Design review of the part built by this model. Coordinates are the model's own, in mm. Face numbers are marked on the shaded views. A direction names the side the tool comes from. Coordinates: 2 decimals unless noted, no trailing zeros. Loops run counter-clockwise (first coordinate to the right, second up) from the corner with the lowest first, then second, coordinate; pieces in that order, holes last. Notation, with made-up numbers: M -13.5,35.25 L 44.5,35.25 A24 ccw 44.5,60.25 Z; hole C 3,-30.5 d9. An arc over 180 degrees is marked long. Answer as a JSON object with one key per item and string values. Group by question number.
1. Draft analysis for pull direction Y (two halves, no side actions). For the marked faces 4, 5 and 6, state which applies: +Y half, -Y half, draft (parallel to the pull), parting line (faces both ways), or undercut.
2. Machinability: for the marked faces 1, 2 and 3, which of the approach directions +Z, -Z, +X, -X, +Y, -Y give a long, thin tool a straight path to every point of the face, cutting with its end or side? Answer none if there is none.
3. Consider section B-B (y = 12.75). State the section outline as (x, z) points, then the cut area to 3 significant figures.
4. Consider section A-A (z = 4.5). State the section outline as (x, y) points.
5. Consider section C-C (x = 11.75). State the section outline as (y, z) points.
6. To check wall thickness, follow probe 1 along Y at (x, z) = (13.25, 3); probe 2 along X at (y, z) = (11.75, 7.75); probe 3 along Z at (x, y) = (16, 2.75). State the ranges of each line that lie inside material, in increasing order.
7. Insertion check: pin 1 (1.5 mm diameter, centred on x = 9, y = 5, fed in from +Z); pin 2 (1.5 mm diameter, centred on x = 10, y = 14, fed in from +Z). Each pin has a flat end and moves straight along its axis. Give the tip position at first contact, or say it passes through.
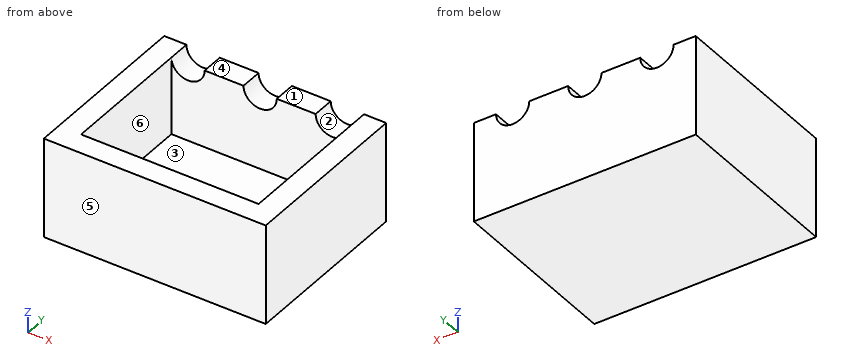
from build123d import *

# Parameters (mm, degrees)
SKETCH1_W           = 20
SKETCH1_H           = 16
BOSS_EXTRUDE1_DEPTH = 9
SKETCH2_W           = 16
SKETCH2_H           = 12
CUT_EXTRUDE1_DEPTH  = 7
SKETCH4_R           = 1.5
CUT_EXTRUDE3_DEPTH  = 7


with BuildPart() as part:
    # Sketch1 → Boss-Extrude1 (new body)
    with BuildSketch(Plane.XY):
        with Locations((10, 8)):
            Rectangle(SKETCH1_W, SKETCH1_H)
    extrude(amount=BOSS_EXTRUDE1_DEPTH)

    # Sketch2 → Cut-Extrude1 (cut)
    with BuildSketch(Plane.XY.offset(9)):
        with Locations((10, 8)):
            Rectangle(SKETCH2_W, SKETCH2_H)
    extrude(amount=-CUT_EXTRUDE1_DEPTH, mode=Mode.SUBTRACT)

    # Sketch4 → Cut-Extrude3 (cut)
    with BuildSketch(Plane(origin=(0, 16, 0), x_dir=(1, 0, 0), z_dir=(0, 1, 0))):
        with Locations((3.5, -9)):
            Circle(SKETCH4_R)
        with Locations((10, -9)):
            Circle(SKETCH4_R)
        with Locations((16.5, -9)):
            Circle(SKETCH4_R)
    extrude(amount=-CUT_EXTRUDE3_DEPTH, mode=Mode.SUBTRACT)


solid = part.part
Findings below:
{
 "1": {"face 4": "draft", "face 5": "-Y half", "face 6": "undercut"},
 "2": {"face 1": "+Z, +X, -X, +Y, -Y", "face 2": "+Z, +Y", "face 3": "+Z"},
 "3": {"outline": "M 0,0 L 20,0 L 20,9 L 18,9 L 18,2 L 2,2 L 2,9 L 0,9 Z", "area": "68.0 mm^2"},
 "4": {"outline": "M 0,0 L 20,0 L 20,16 L 0,16 Z; hole M 2,2 L 18,2 L 18,14 L 2,14 Z"},
 "5": {"outline": "M 0,0 L 16,0 L 16,9 L 14,9 L 14,2 L 2,2 L 2,9 L 0,9 Z"},
 "6": {"probe 1": "y = 0 to 2, 14 to 16", "probe 2": "x = 0 to 2, 18 to 20", "probe 3": "z = 0 to 2"},
 "7": {"pin 1": "stops at z = 2", "pin 2": "stops at z = 7.7"}
}
